```python
from build123d import *

# Parameters (mm, degrees)
SKETCH1_W           = 120.4
SKETCH1_H           = 76.28
BOSS_EXTRUDE1_DEPTH = 24
FILLET1_R           = 9.5
SKETCH2_R           = 1.5
CUT_EXTRUDE1_DEPTH  = 22


with BuildPart() as part:
    # Sketch1 → Boss-Extrude1 (new body)
    with BuildSketch(Plane(origin=(0, 0, 0), x_dir=(1, 0, 0), z_dir=(0, 1, 0))):
        Rectangle(SKETCH1_W, SKETCH1_H)
    extrude(amount=BOSS_EXTRUDE1_DEPTH)

    # Fillet1
    fillet1_edges = [part.edges().sort_by_distance(p)[0] for p in [
        (60.2, 12, 38.14),
        (-60.2, 12, 38.14),
        (-60.2, 12, -38.14),
        (60.2, 12, -38.14),
    ]]
    fillet(fillet1_edges, radius=FILLET1_R)

    # Sketch2 → Cut-Extrude1 (cut)
    with BuildSketch(Plane(origin=(0, 24, 0), x_dir=(1, 0, 0), z_dir=(0, 1, 0))):
        with Locations(Location((50.57, -28.51, 0), (0, 0, 270))):
            Circle(SKETCH2_R)
        with Locations(Location((50.57, 28.51, 0), (0, 0, 90))):
            Circle(SKETCH2_R)
        with BuildLine():
            Line((-49.2, 36.64), (-5.840999167, 36.64))
            ThreePointArc((-5.840999167, 36.64), (-5.133892386, 36.347106781), (-4.840999167, 35.64))
            Line((-4.840999167, 35.64), (-4.840999167, 34.772736938))
            ThreePointArc((-4.840999167, 34.772736938), (-4.548105948, 34.065630157), (-3.840999167, 33.772736938))
            Line((-3.840999167, 33.772736938), (0.159000833, 33.772736938))
            ThreePointArc((0.159000833, 33.772736938), (0.866107614, 34.065630157), (1.159000833, 34.772736938))
            Line((1.159000833, 34.772736938), (1.159000833, 35.64))
            ThreePointArc((1.159000833, 35.64), (1.451894052, 36.347106781), (2.159000833, 36.64))
            Line((2.159000833, 36.64), (36.94, 36.64))
            ThreePointArc((36.94, 36.64), (40.829087297, 35.029087297), (42.44, 31.14))
            Line((42.44, 31.14), (42.44, 28.51))
            ThreePointArc((42.44, 28.51), (44.821221869, 22.761221869), (50.57, 20.38))
            Line((50.57, 20.38), (53.2, 20.38))
            ThreePointArc((53.2, 20.38), (57.089087297, 18.769087297), (58.7, 14.88))
            Line((58.7, 14.88), (58.7, -14.88))
            ThreePointArc((58.7, -14.88), (57.089087297, -18.769087297), (53.2, -20.38))
            Line((53.2, -20.38), (50.57, -20.38))
            ThreePointArc((50.57, -20.38), (44.821221869, -22.761221869), (42.44, -28.51))
            Line((42.44, -28.51), (42.44, -31.14))
            ThreePointArc((42.44, -31.14), (40.829087297, -35.029087297), (36.94, -36.64))
            Line((36.94, -36.64), (2.159000833, -36.64))
            ThreePointArc((2.159000833, -36.64), (1.451894052, -36.347106781), (1.159000833, -35.64))
            Line((1.159000833, -35.64), (1.159000833, -34.772736938))
            ThreePointArc((1.159000833, -34.772736938), (0.866107614, -34.065630157), (0.159000833, -33.772736938))
            Line((0.159000833, -33.772736938), (-3.840999167, -33.772736938))
            ThreePointArc((-3.840999167, -33.772736938), (-4.548105948, -34.065630157), (-4.840999167, -34.772736938))
            Line((-4.840999167, -34.772736938), (-4.840999167, -35.64))
            ThreePointArc((-4.840999167, -35.64), (-5.133892386, -36.347106781), (-5.840999167, -36.64))
            Line((-5.840999167, -36.64), (-49.2, -36.64))
            ThreePointArc((-49.2, -36.64), (-55.917514421, -33.857514421), (-58.7, -27.14))
            Line((-58.7, -27.14), (-58.7, 27.14))
            ThreePointArc((-58.7, 27.14), (-55.917514421, 33.857514421), (-49.2, 36.64))
        make_face()
    extrude(amount=-CUT_EXTRUDE1_DEPTH, mode=Mode.SUBTRACT)


solid = part.part
```
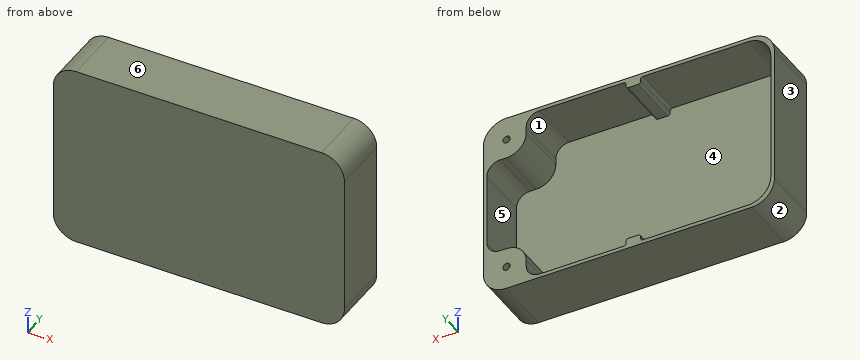
Geometry check sheet. Reference: the model listing, model coordinates, mm. Face numbers are marked on the shaded views. A direction names the side the tool comes from. Give positions to 0.01 mm unless a question says otherwise; leave off trailing zeros. Write each loop counter-clockwise with the first axis right and the second up, starting at its lowest first coordinate (ties: lowest second). Pieces come first, ordered by that corner, then holes.
1) Section check A-A, the plane z = -10. Record the boundary of the cut face in (x, y).
2) Gauge pin test, flat ends, axial feed: pin 1 (1.8 mm diameter, centred on x = 50.57, z = -28.51, fed in from -Y); pin 2 (3 mm diameter, centred on x = 23.5, z = 18, fed in from +Y); pin 3 (1 mm diameter, centred on y = 11, z = 35, fed in from +X); pin 4 (0.7 mm diameter, centred on y = 17, z = 35.5, fed in from -X). Record the tip position at first contact, or that the pin passes through.
3) Section check C-C, the plane y = 14.5. State how many separate pieces and enclosed holes the cut face has, and give its area (3 significant figures).
4) Release check for a two-part mould opening along X. For the marked faces 3, 4, 5 and 6 record: pulls with the +X half, pulls with the -X half, needs draft (parallel to the pull), parting line crosses it, or undercut.
5) Section check B-B, the plane x = -25. Record the boundary of the cut face in (y, z).
6) Access from +Z, -Z, +X, -X, +Y, -Y to the whole of each face (thin tool, end or side, straight path). Record for the marked faces 1 and 2.
7) Material ranges on L1, parallel to Z at x = 0, y = 3.5; L2, parallel to Z at x = -33, y = 2.5; L3, parallel to X at y = 19, z = -29.5, recorded low to high.
Computed:
1. outline: (-60.2, 0) - (60.2, 0) - (60.2, 24) - (58.7, 24) - (58.7, 2) - (-58.7, 2) - (-58.7, 24) - (-60.2, 24) - close
2. pin 1: stops at y = 0
2. pin 2: stops at y = 2
2. pin 3: stops at x = 58.18
2. pin 4: stops at x = -57.62
3. separate pieces: 1
3. enclosed holes: 3
3. area: 1,090 mm2
4. face 3: pulls with the -X half
4. face 4: undercut
4. face 5: undercut
4. face 6: needs draft
5. outline: (0, -38.14) - (24, -38.14) - (24, -36.64) - (2, -36.64) - (2, 36.64) - (24, 36.64) - (24, 38.14) - (0, 38.14) - close
6. face 1: +Y
6. face 2: -Z, -X, +Y, -Y
7. L1: z = -38.14 to -33.77, 33.77 to 38.14
7. L2: z = -38.14 to -36.64, 36.64 to 38.14
7. L3: x = -60.16 to -58.4, 42.44 to 49.44, 51.7 to 60.16
